Here's how the part is built. I have some questions about the finished solid (model axes, mm). A direction names the side the tool comes from. Give positions to 0.01 mm unless a question says otherwise; leave off trailing zeros. Order: outer loops, then holes, each group sorted by start corner. A loop starts at its lowest first (then second) coordinate and runs counter-clockwise, first axis right, second up. Notation, with made-up numbers: (86.5, 18) -> (128.5, 18) arc R21 ccw to (128.5, 26) -> close; hole circle Ø7 at (82.5, 30). An arc over 180 degrees is marked (long way). Write each question's results on one line, items separated by ' | '. Start each with the question number.
Q1. Imagine slicing it at A-A, the plane x = 30.49. Please give me the cut outline in (y, z).
Q2. I'm going to push a flat-ended pin straight in: pin 1 (1.7 mm diameter, centred on x = 31, y = 5, fed in from +Z). Where does the tip first touch, or does it pass through?
Q3. For faces 4 (the face through (28.77, 5.17, 0.99)), 5 (the face through (35.721, 19.335, 0.479)), which set-ups out of +Z, -Z, +X, -X, +Y, -Y let a thin tool reach every point of the face, with its end or its side?
Q4. Imagine slicing it at B-B, the plane y = 5.09. Please give me the cut outline in (x, z), then the cut area to 3 significant figures.
Q5. Thinking about a two-plate mould opening in X: for faces 1 (the face through (18, 10, -1)), 2 (the face through (30, 5, 0)), 3 (the face through (35.735, 0.259, 0.521)), which applies, pulls with the +X half, pulls with the -X half, needs draft (parallel to the pull), parting line crosses it, or undercut?
Q6. I need wall thicknesses on line 1 along Y through (x, z) = (30.49, 0.5); line 2 along Y through (x, z) = (31, 0.4); line 3 along X through (y, z) = (6, 1.8). Which ranges of each line are inside material? Lowest first, please. Write a range as [from, to].
```python
from build123d import *

# Parameters (mm, degrees)
SKETCH_W     = 35.98
SKETCH_H     = 19.58
SKETCH_R     = 1.72
PAD_DEPTH    = 2
SKETCH001_W  = 35.98
SKETCH001_H  = 19.58
PAD001_DEPTH = 1
FILLET_R     = 0.86


with BuildPart() as part:
    # Sketch → Pad (new body)
    with BuildSketch(Plane.XY):
        with Locations((17.99, 9.79)):
            Rectangle(SKETCH_W, SKETCH_H)
        with Locations((30.49, 5.09)):
            Circle(SKETCH_R, mode=Mode.SUBTRACT)
    extrude(amount=PAD_DEPTH)

    # Sketch001 (on Face6 of Pad) → Pad001 (join)
    with BuildSketch(Plane(origin=(0, 0, 0), x_dir=(1, 0, 0), z_dir=(0, 0, -1))):
        with Locations((17.99, -9.79)):
            Rectangle(SKETCH001_W, SKETCH001_H)
    extrude(amount=PAD001_DEPTH)

    # Fillet
    fillet_edges = [part.edges().sort_by_distance(p)[0] for p in [
        (0, 0, 0.5),
        (0, 19.58, 0.5),
        (35.98, 19.58, 0.5),
        (35.98, 0, 0.5),
    ]]
    fillet(fillet_edges, radius=FILLET_R)


solid = part.part
```
Geometry check:
1) outline: (0, -1) -> (19.58, -1) -> (19.58, 2) -> (6.81, 2) -> (6.81, 0) -> (3.37, 0) -> (3.37, 2) -> (0, 2) -> close
2) pin 1: z = 0
3) face 4: +Z | face 5: +Z, -Z, +X, +Y
4) outline: (0, -1) -> (35.98, -1) -> (35.98, 2) -> (32.21, 2) -> (32.21, 0) -> (28.77, 0) -> (28.77, 2) -> (0, 2) -> close | area: 101 mm²
5) face 1: needs draft | face 2: undercut | face 3: pulls with the +X half
6) line 1: [0, 3.37], [6.81, 19.58] | line 2: [0, 3.45], [6.73, 19.58] | line 3: [0, 29.03], [31.95, 35.98]
